Verification items for this drawing (mm, ordinates from the low corner). A direction names the side the tool comes from. Round coordinates to 2 decimals unless told otherwise and drop trailing zeros. Order: outer loops, then holes, each group sorted by start corner. A loop starts at its lowest first (then second) coordinate and runs counter-clockwise, first axis right, second up. Notation, with made-up numbers: (-32.75, -4) -> (0.25, -4) arc R14 cw to (0.25, 16) -> close; hole circle Ø5 at (84, 36). An arc over 180 degrees is marked (long way). Answer in a Markdown table with one row per item. Add a question column.
1. Access from +Z, -Z, +X, -X, +Y, -Y to the whole of each face (thin tool, end or side, straight path). Record for the marked faces 1 and 2.
2. Sectioned sample at C-C, the plane z = 36.5. Record the boundary of the cut face in (x, y), then the cut area to 3 significant figures.
3. Sectioned sample at B-B, the plane x = 43. Record the boundary of the cut face in (y, z).
4. Material ranges on L1, parallel to Z at x = 42.5, y = 9; L2, parallel to X at y = 8, z = 22; L3, parallel to Y at x = 62, z = 19, recorded low to high. Write a range as from..to.
5. Sectioned sample at A-A, the plane y = 3.5. Record the boundary of the cut face in (x, z), then the cut area to 3 significant figures.
6. Draft check along X on the marked faces 3, 4 and 5. Enter one of: +X half, -X half, draft (parallel to the pull), parting line (faces both ways), or undercut.
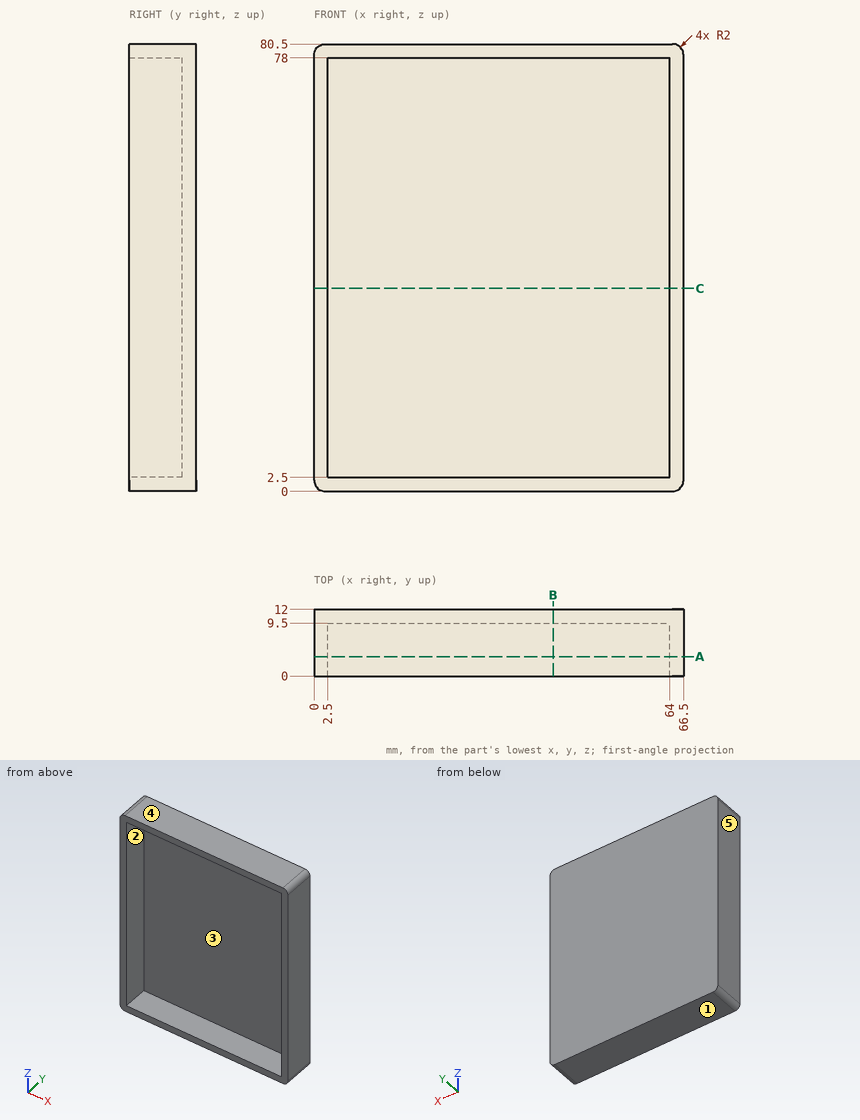
Answer key:
| question | item | result |
|---|---|---|
| 1 | face 1 | -Z, +X, -X, +Y, -Y |
| 1 | face 2 | -Y |
| 2 | outline | (0, 0) -> (2.5, 0) -> (2.5, 9.5) -> (64, 9.5) -> (64, 0) -> (66.5, 0) -> (66.5, 12) -> (0, 12) -> close |
| 2 | area | 214 mm² |
| 3 | outline | (0, 0) -> (12, 0) -> (12, 80.5) -> (0, 80.5) -> (0, 78) -> (9.5, 78) -> (9.5, 2.5) -> (0, 2.5) -> close |
| 4 | L1 | z = 0..2.5, 78..80.5 |
| 4 | L2 | x = 0..2.5, 64..66.5 |
| 4 | L3 | y = 9.5..12 |
| 5 | outline | (0, 2) arc R2 ccw to (2, 0) -> (64.5, 0) arc R2 ccw to (66.5, 2) -> (66.5, 78.5) arc R2 ccw to (64.5, 80.5) -> (2, 80.5) arc R2 ccw to (0, 78.5) -> close; hole (2.5, 2.5) -> (64, 2.5) -> (64, 78) -> (2.5, 78) -> close |
| 5 | area | 707 mm² |
| 6 | face 3 | undercut |
| 6 | face 4 | draft |
| 6 | face 5 | -X half |
